```python
from build123d import *

# Parameters (mm, degrees)
SKETCH1_R           = 3.96875
SKETCH1_R_2         = 3.175
BOSS_EXTRUDE1_DEPTH = 10.16
CUT_EXTRUDE1_DEPTH  = 5.08


with BuildPart() as part:
    # Sketch1 → Boss-Extrude1 (new body)
    with BuildSketch(Plane(origin=(0, 0, 0), x_dir=(1, 0, 0), z_dir=(0, 1, 0))):
        with BuildLine():
            Line((38.1, -5.08), (6.098975836, -5.08))
            ThreePointArc((6.098975836, -5.08), (-2.701229863, -7.463729863), (-7.9375, 0))
            Line((-7.9375, 0), (-12.3825, 13.97))
            Line((-12.3825, 13.97), (-12.3825, 31.75))
            Line((-12.3825, 31.75), (54.2925, 31.75))
            Line((54.2925, 31.75), (54.2925, 13.97))
            Line((54.2925, 13.97), (48.26, 0))
            ThreePointArc((48.26, 0), (44.749806331, -5.679612663), (38.1, -5.08))
        make_face()
        with Locations(Location((0, 0, 0), (0, 0, 270))):
            Circle(SKETCH1_R, mode=Mode.SUBTRACT)
        with Locations(Location((41.91, 0, 0), (0, 0, 270))):
            Circle(SKETCH1_R_2, mode=Mode.SUBTRACT)
        with Locations(Location((46.355, 22.86, 0), (0, 0, 270))):
            Circle(SKETCH1_R, mode=Mode.SUBTRACT)
        with Locations(Location((-4.445, 22.86, 0), (0, 0, 270))):
            Circle(SKETCH1_R, mode=Mode.SUBTRACT)
        with BuildLine():
            Line((17.139504023, -0.186733089), (14.878562514, 3.04222602))
            ThreePointArc((14.878562514, 3.04222602), (11.369192259, -1.821105185), (17.139504023, -0.186733089))
        make_face(mode=Mode.SUBTRACT)
    extrude(amount=-BOSS_EXTRUDE1_DEPTH)

    # Sketch2 → Cut-Extrude1 (cut)
    with BuildSketch(Plane.XZ.offset(10.16)):
        with BuildLine():
            Line((9.2075, 0), (9.2075, 5.08))
            Line((9.2075, 5.08), (18.7325, 5.08))
            Line((18.7325, 5.08), (18.7325, 0))
            ThreePointArc((18.7325, 0), (13.97, -4.7625), (9.2075, 0))
        make_face()
    extrude(amount=-CUT_EXTRUDE1_DEPTH, mode=Mode.SUBTRACT)


solid = part.part
```
Input: part model. Units: mm. Frame: model coordinates. A direction names the side the tool comes from. Round coordinates to 2 decimals unless told otherwise and drop trailing zeros. Order: outer loops, then holes, each group sorted by start corner. A loop starts at its lowest first (then second) coordinate and runs counter-clockwise, first axis right, second up. Notation, with made-up numbers: (42.5, -9.75) - (68.5, -9.75) arc R24 cw to (68.5, 18.25) - close; hole circle Ø9 at (2, 88.25). An arc over 180 degrees is marked (long way). One line per question, with ' | ' between items. Start each with the question number.
1) Contact query for flat-ended pins moving along their axis: P1, Ø4, axis at y = -8.5, z = 3.5, coming from the +X side; P2, Ø1.5, axis at y = -8, z = -12.5, coming from the +X side; P3, Ø2.5, axis at y = -8, z = 2.5, coming from the -X side. Output: stop coordinate, or through.
2) Cut plane D-D, the plane z = -1. Return the cut outline in (x, y), then the cut area to 3 significant figures.
3) Pull-direction query (X, two-part tool) for faces 1 (the flat face through (-12.382, -5, -23)), 2 (the cylindrical face through (42.48, -5.01, -23.72)), 3 (the flat face through (51.318, -5.009, -7.083)); classes: +X half, -X half, draft (parallel to the pull), parting line (faces both ways), or undercut.
4) Ray query, probe 1 along X at (y, z) = (-5.25, -22.86); probe 2 along X at (y, z) = (-2.75, 0) (1 decimal); probe 3 along X at (y, z) = (-3, 2). Return the intervals inside material, ascending.
5) Cut plane A-A, the plane z = -22.86. Return the cut outline in (x, y), then the cut area to 3 significant figures.
6) Set-up query: faces 4 (the flat face through (16.02, -2.5, -1.41)), 5 (the flat face through (-10.13, -5.01, -6.89)), 6 (the flat face through (9.208, -8, 3)), 7 (the flat face through (20, -5, -31.75)), 8 (the flat face through (22, -5, 5.08)). Return all of +Z, -Z, +X, -X, +Y, -Y with unobstructed straight access to the full face (end or side cutting, diameter ignored); none if empty.
7) Cut plane C-C, the plane y = -6.5. Give the number of separate pieces and of enclosed holes in the cut face, then the cut area to 3 significant figures.
Worked out:
1) P1: stops at x = 48.08 | P2: stops at x = 53.98 | P3: stops at x = -7.84
2) outline: (-8.26, -10.16) - (-3.84, -10.16) - (-3.84, 0) - (-8.26, 0) - close; (3.84, -10.16) - (9.31, -10.16) - (9.31, -5.08) - (10.96, -5.08) - (10.96, 0) - (3.84, 0) - close; (16.31, -5.08) - (18.63, -5.08) - (18.63, -10.16) - (38.9, -10.16) - (38.9, 0) - (16.31, 0) - close; (44.92, -10.16) - (48.69, -10.16) - (48.69, 0) - (44.92, 0) - close | area: 365 mm^2
3) face 1: -X half | face 2: undercut | face 3: +X half
4) probe 1: x = -12.38 to -8.41, -0.48 to 42.39, 50.32 to 54.29 | probe 2: x = -7.9 to -4, 4 to 10.8, 17 to 38.7, 45.1 to 48.3 | probe 3: x = -7.68 to -3.43, 3.43 to 11.5, 16.44 to 39.44, 44.38 to 47.94
5) outline: (-12.38, -10.16) - (-8.41, -10.16) - (-8.41, 0) - (-12.38, 0) - close; (-0.48, -10.16) - (42.39, -10.16) - (42.39, 0) - (-0.48, 0) - close; (50.32, -10.16) - (54.29, -10.16) - (54.29, 0) - (50.32, 0) - close | area: 516 mm^2
6) face 4: +Y, -Y | face 5: +Z, -X, +Y, -Y | face 6: +Z, -Y | face 7: -Z, +X, -X, +Y, -Y | face 8: +Z, +Y, -Y
7) separate pieces: 1 | enclosed holes: 4 | area: 2,090 mm^2
